Read the model definition and answer for the solid it produces. Units are mm, in the model's axes. Coordinates: 2 decimals unless noted, no trailing zeros. Order: outer loops, then holes, each group sorted by start corner. A loop starts at its lowest first (then second) coordinate and runs counter-clockwise, first axis right, second up. Notation, with made-up numbers: (87, 77) - (92, 77) arc R18 ccw to (92, 104) - close; hole circle Ø2 at (74.25, -26). An arc over 180 degrees is marked (long way). Use one line per item in the form item = value.
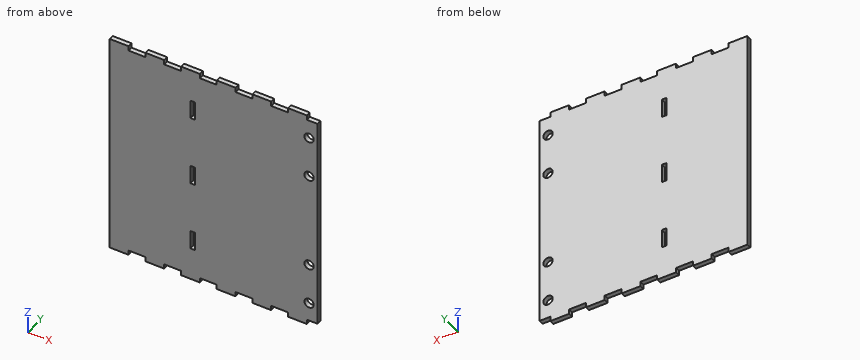
```python
from build123d import *

# Parameters (mm, degrees)
BOSS_EXTRUDE1_DEPTH = 6.35
SKETCH2_R           = 6.35
SKETCH2_W           = 6.35
SKETCH2_H           = 25.4
CUT_EXTRUDE1_DEPTH  = 340.756694235


with BuildPart() as part:
    # Sketch1 → Boss-Extrude1 (new body)
    with BuildSketch(Plane(origin=(0, 0, 0), x_dir=(1, 0, 0), z_dir=(0, 1, 0))):
        Polygon((-97.696931278, -1.942339741), (-72.296931278, -1.942339741), (-72.296931278, -8.292339741), (-49.436931278, -8.292339741), (-49.436931278, -1.942339741), (-24.036931278, -1.942339741), (-24.036931278, -8.292339741), (-1.176931278, -8.292339741), (-1.176931278, -1.942339741), (24.223068722, -1.942339741), (24.223068722, -8.292339741), (47.083068722, -8.292339741), (47.083068722, -1.942339741), (72.483068722, -1.942339741), (72.483068722, -8.292339741), (95.343068722, -8.292339741), (95.343068722, -1.942339741), (120.743068722, -1.942339741), (120.743068722, -8.292339741), (134.967068722, -8.292339741), (134.967068722, -300.392339741), (120.743068722, -300.392339741), (120.743068722, -306.742339741), (95.343068722, -306.742339741), (95.343068722, -300.392339741), (72.483068722, -300.392339741), (72.483068722, -306.742339741), (47.083068722, -306.742339741), (47.083068722, -300.392339741), (24.223068722, -300.392339741), (24.223068722, -306.742339741), (-1.176931278, -306.742339741), (-1.176931278, -300.392339741), (-24.036931278, -300.392339741), (-24.036931278, -306.742339741), (-49.436931278, -306.742339741), (-49.436931278, -300.392339741), (-72.296931278, -300.392339741), (-72.296931278, -306.742339741), (-97.696931278, -306.742339741), (-97.696931278, -300.392339741), (-120.556931278, -300.392339741), (-120.556931278, -306.742339741), (-145.956931278, -306.742339741), (-145.956931278, -300.392339741), (-145.956931278, -8.292339741), (-145.956931278, -1.942339741), (-120.556931278, -1.942339741), (-120.556931278, -8.292339741), (-97.696931278, -8.292339741), align=None)
    extrude(amount=BOSS_EXTRUDE1_DEPTH)

    # Sketch2 → Cut-Extrude1 (cut, through all)
    with BuildSketch(Plane(origin=(0, 6.35, 0), x_dir=(1, 0, 0), z_dir=(0, 1, 0))):
        with Locations(Location((123.791068722, -274.992339741, 0), (0, 0, 270))):
            Circle(SKETCH2_R)
        with Locations(Location((123.791068722, -33.692339741, 0), (0, 0, 270))):
            Circle(SKETCH2_R)
        with Locations(Location((123.791068722, -89.572339741, 0), (0, 0, 270))):
            Circle(SKETCH2_R)
        with Locations(Location((123.791068722, -219.112339741, 0), (0, 0, 270))):
            Circle(SKETCH2_R)
        with Locations((-33.561931278, -59.092339741)):
            Rectangle(SKETCH2_W, SKETCH2_H)
        with Locations((-33.561931278, -249.592339741)):
            Rectangle(SKETCH2_W, SKETCH2_H)
        with Locations((-33.561931278, -154.342339741)):
            Rectangle(SKETCH2_W, SKETCH2_H)
    extrude(amount=-CUT_EXTRUDE1_DEPTH, mode=Mode.SUBTRACT)


solid = part.part
```
(1) Straight lines are drawn through the part: L1, parallel to X at y = 5.75, z = 243; L2, parallel to X at y = 2, z = 35.5; L3, parallel to Z at x = -117.5, y = 5.75. For each, find the intervals that lie inside material, in ascending order.
Answer list:
L1 = -145.96 to -36.74, -30.39 to 134.97
L2 = -145.96 to 117.7, 129.88 to 134.97
L3 = 8.29 to 300.39
(2) Section B-B, the plane y = 2.75 is taken. State how many separate pieces and enclosed holes the cut face has, then the cut area to 3 significant figures.
Answer list:
separate_pieces = 1
enclosed_holes = 7
area = 83,000 mm2
(3) Given pin 1 Ø1.9 at (y, z) = (4, 302.5) entering from +X; pin 2 Ø3 at (x, y) = (-56, 4) entering from -Z, each flat-ended and moving along its own axis, determine where each tip first touches the part or whether it passes through.
Answer list:
pin_1 = 120.74
pin_2 = 8.29
(4) Section A-A, the plane x = -62.5 is taken. Write down the section's boundary in (y, z), then the cut area to 3 significant figures.
Answer list:
outline = (0, 8.29) - (6.35, 8.29) - (6.35, 300.39) - (0, 300.39) - close
area = 1,850 mm2
